Can you work these out from the model? Positions are in its coordinate system, mm. A direction names the side the tool comes from. Give positions to 0.01 mm unless a question says otherwise; leave off trailing zeros. Answer as CSV lines item,"result".
```python
from build123d import *

# Parameters (mm, degrees)
F1_DEPTH  = 6.35
F2_DEPTH  = 3.175
F3_DEPTH  = 2.8222222222
F4_DEPTH  = 2.4694444444
F5_DEPTH  = 2.4694444444
F6_DEPTH  = 2.1166666667
F7_DEPTH  = 1.4111111111
F8_DEPTH  = 1.0583333333
F9_DEPTH  = 0.3527777778
F10_DEPTH = 0.7055555556
F12_DEPTH = 2.54
F13_R     = 2.38125
F14_DEPTH = 25.4
F15_R     = 2.53999
F16_R     = 2.53999
F18_DEPTH = 2.54


# Not quite as in the source:
# - a fillet or chamfer is up to 0.001 mm smaller than in the source, because OpenCascade refuses the exact size


with BuildPart() as f1:
    # F0 (on Top) → F1 (new body)
    with BuildSketch(Plane.XY):
        Polygon((152.4, 3.6661742094), (152.4, 0), (152.4, -3.6661742094), (158.75, -7.3323484187), (165.1, -3.6661742094), (165.1, 3.6661742094), (158.75, 7.3323484187), align=None)
    extrude(amount=F1_DEPTH)

    # F6 (add): a face of the model
    f6_faces = [f1.faces().sort_by_distance(p)[0] for p in [
        (158.75, 0, 6.35),
    ]]
    extrude(f6_faces, amount=F6_DEPTH)


with BuildPart() as f1b:
    # F0 (on Top) → F1, piece 2 (new body)
    with BuildSketch(Plane.XY):
        Polygon((144.4625, -36.2669128953), (141.2875, -34.4338257906), (138.1125, -36.2669128953), (138.1125, -39.9330871047), (141.2875, -41.7661742094), (144.4625, -39.9330871047), align=None)
    extrude(amount=F1_DEPTH)


with BuildPart() as f1c:
    # F0 (on Top) → F1, piece 3 (new body)
    with BuildSketch(Plane.XY):
        Polygon((116.68125, 4.1244459855), (116.68125, 0), (123.825, 0), (130.96875, 0), (130.96875, 4.1244459855), (123.825, 8.248891971), align=None)
        Polygon((123.825, 0), (116.68125, 0), (116.68125, -4.1244459855), (123.825, -8.248891971), (130.96875, -4.1244459855), (130.96875, 0), align=None)
    extrude(amount=F1_DEPTH)

    # F5 (add): a face of the model
    f5_faces = [f1c.faces().sort_by_distance(p)[0] for p in [
        (123.825, 0, 6.35),
    ]]
    extrude(f5_faces, amount=F5_DEPTH)


with BuildPart() as f1d:
    # F0 (on Top) → F1, piece 4 (new body)
    with BuildSketch(Plane.XY):
        Polygon((108.74375, -35.8086411192), (104.775, -33.5172822383), (100.80625, -35.8086411192), (100.80625, -40.3913588808), (104.775, -42.6827177617), (108.74375, -40.3913588808), align=None)
    extrude(amount=F1_DEPTH)

    # F9 (add): a face of the model
    f9_faces = [f1d.faces().sort_by_distance(p)[0] for p in [
        (104.775, -38.1, 6.35),
    ]]
    extrude(f9_faces, amount=F9_DEPTH)


with BuildPart() as f1e:
    # F0 (on Top) → F1, piece 5 (new body)
    with BuildSketch(Plane.XY):
        Polygon((77.7875, 4.5827177617), (77.7875, 0), (85.725, 0), (93.6625, 0), (93.6625, 4.5827177617), (85.725, 9.1654355234), align=None)
        Polygon((85.725, 0), (77.7875, 0), (77.7875, -4.5827177617), (85.725, -9.1654355234), (93.6625, -4.5827177617), (93.6625, 0), align=None)
    extrude(amount=F1_DEPTH)

    # F4 (add): a face of the model
    f4_faces = [f1e.faces().sort_by_distance(p)[0] for p in [
        (85.725, 0, 6.35),
    ]]
    extrude(f4_faces, amount=F4_DEPTH)


with BuildPart() as f1f:
    # F0 (on Top) → F1, piece 6 (new body)
    with BuildSketch(Plane.XY):
        Polygon((69.453125, -35.5795052311), (65.0875, -33.0590104621), (60.721875, -35.5795052311), (60.721875, -40.6204947689), (65.0875, -43.1409895379), (69.453125, -40.6204947689), align=None)
    extrude(amount=F1_DEPTH)

    # F10 (add): a face of the model
    f10_faces = [f1f.faces().sort_by_distance(p)[0] for p in [
        (65.0875, -38.1, 6.35),
    ]]
    extrude(f10_faces, amount=F10_DEPTH)


with BuildPart() as f1g:
    # F0 (on Top) → F1, piece 7 (new body)
    with BuildSketch(Plane.XY):
        Polygon((35.71875, 5.0409895379), (35.71875, 0), (44.45, 0), (53.18125, 0), (53.18125, 5.0409895379), (44.45, 10.0819790757), align=None)
        Polygon((44.45, 0), (35.71875, 0), (35.71875, -5.0409895379), (44.45, -10.0819790757), (53.18125, -5.0409895379), (53.18125, 0), align=None)
    extrude(amount=F1_DEPTH)

    # F3 (add): a face of the model
    f3_faces = [f1g.faces().sort_by_distance(p)[0] for p in [
        (44.45, 0, 6.35),
    ]]
    extrude(f3_faces, amount=F3_DEPTH)


with BuildPart() as f1h:
    # F0 (on Top) → F1, piece 8 (new body)
    with BuildSketch(Plane.XY):
        Polygon((-18.25625, -41.3079024332), (-18.25625, -38.1), (-18.25625, -34.8920975668), (-23.8125, -31.6841951336), (-29.36875, -34.8920975668), (-29.36875, -41.3079024332), (-23.8125, -44.5158048664), align=None)
    extrude(amount=F1_DEPTH)

    # F7 (add): a face of the model
    f7_faces = [f1h.faces().sort_by_distance(p)[0] for p in [
        (-23.8125, -38.1, 6.35),
    ]]
    extrude(f7_faces, amount=F7_DEPTH)


with BuildPart() as f1i:
    # F0 (on Top) → F1, piece 9 (new body)
    with BuildSketch(Plane.XY):
        Polygon((26.9875, -35.350369343), (22.225, -32.600738686), (22.225, -38.1), (17.4625, -38.1), (17.4625, -40.849630657), (22.225, -43.599261314), (26.9875, -40.849630657), align=None)
        Polygon((22.225, -38.1), (22.225, -32.600738686), (17.4625, -35.350369343), (17.4625, -38.1), align=None)
    extrude(amount=F1_DEPTH)

    # F8 (add): a face of the model
    f8_faces = [f1i.faces().sort_by_distance(p)[0] for p in [
        (22.225, -38.1, 6.35),
    ]]
    extrude(f8_faces, amount=F8_DEPTH)


with BuildPart() as f1j:
    # F0 (on Top) → F1, piece 10 (new body)
    with BuildSketch(Plane.XY):
        Polygon((9.525, -5.499261314), (9.525, 0), (9.525, 5.499261314), (0, 10.9985226281), (-9.525, 5.499261314), (-9.525, -5.499261314), (0, -10.9985226281), align=None)
    extrude(amount=F1_DEPTH)

    # F2 (add): a face of the model
    f2_faces = [f1j.faces().sort_by_distance(p)[0] for p in [
        (0, 0, 6.35),
    ]]
    extrude(f2_faces, amount=F2_DEPTH)


with BuildPart() as f12:
    # F11 (on face) → F12 (new body)
    with BuildSketch(Plane(origin=(0, 0, 0), x_dir=(1, 0, 0), z_dir=(0, 0, -1))):
        with BuildLine():
            Line((141.2875, 47.6267617683), (-23.5682692308, 50.7976514101))
            ThreePointArc((-23.5682692308, 50.7976514101), (-14.7463064556, 46.9934883266), (-11.1125, 38.1))
            Line((-11.1125, 38.1), (131.7625, 38.1))
            ThreePointArc((131.7625, 38.1), (134.617383755, 44.8996451583), (141.4706730769, 47.6232385575))
            Line((141.4706730769, 47.6232385575), (141.2875, 47.6267617683))
        make_face()
        with BuildLine():
            Line((-35.4252854215, 32.9586757782), (-17.4191781323, -7.7119863327))
            ThreePointArc((-17.4191781323, -7.7119863327), (-10.2318580693, -16.0689632662), (0.381, -19.0461896189))
            ThreePointArc((0.381, -19.0461896189), (13.6044211564, -13.335), (19.05, 0))
            Line((19.05, 0), (142.875, 0))
            ThreePointArc((142.875, 0), (147.6375, -11.3370176303), (159.0675, -15.8718246824))
            ThreePointArc((159.0675, -15.8718246824), (172.7981495603, -7.3935863375), (172.0126501051, 8.7245479648))
            Line((172.0126501051, 8.7245479648), (149.245090063, 43.3347287789))
            ThreePointArc((149.245090063, 43.3347287789), (145.8881342123, 46.4402511859), (141.4706730769, 47.6232385575))
            ThreePointArc((141.4706730769, 47.6232385575), (134.617383755, 44.8996451583), (131.7625, 38.1))
            Line((131.7625, 38.1), (-11.1125, 38.1))
            ThreePointArc((-11.1125, 38.1), (-14.7463064556, 46.9934883266), (-23.5682692308, 50.7976514101))
            ThreePointArc((-23.5682692308, 50.7976514101), (-34.3892798322, 45.1300589173), (-35.4252854215, 32.9586757782))
        make_face()
        Polygon((9.525, 5.499261314), (9.525, 0), (9.525, -5.499261314), (0, -10.9985226281), (-9.525, -5.499261314), (-9.525, 5.499261314), (0, 10.9985226281), align=None, mode=Mode.SUBTRACT)
        with BuildLine():
            ThreePointArc((19.05, 0), (13.6044211564, -13.335), (0.381, -19.0461896189))
            Line((0.381, -19.0461896189), (159.0675, -15.8718246824))
            ThreePointArc((159.0675, -15.8718246824), (147.6375, -11.3370176303), (142.875, 0))
            Line((142.875, 0), (19.05, 0))
        make_face()
    extrude(amount=F12_DEPTH)

    # F13 (on face) → F14 (cut)
    with BuildSketch(Plane(origin=(0, 0, -2.54), x_dir=(1, 0, 0), z_dir=(0, 0, -1))):
        with Locations((22.225, 19.900738686)):
            Circle(F13_R)
        with Locations((123.825, 19.900738686)):
            Circle(F13_R)
    extrude(amount=-F14_DEPTH, mode=Mode.SUBTRACT)

    # F15 (radius 2.54 in the source; OpenCascade refuses exactly that, so slightly less here)
    f15_edges = [f12.edges().sort_by_distance(p)[0] for p in [
        (19.84375, -19.900739, 0),
    ]]
    fillet(f15_edges, radius=F15_R)

    # F16 (radius 2.54 in the source; OpenCascade refuses exactly that, so slightly less here)
    f16_edges = [f12.edges().sort_by_distance(p)[0] for p in [
        (58.951202, -49.210445, 0),
        (121.44375, -19.900739, 0),
    ]]
    fillet(f16_edges, radius=F16_R)


with BuildPart() as f1j_1:
    add(f1j.part)

    # F17: union F1g, F1e, F1c, F1, F1h, F1i, F1f, F1d, F1b, F12
    add(f1g.part)
    add(f1e.part)
    add(f1c.part)
    add(f1.part)
    add(f1h.part)
    add(f1i.part)
    add(f1f.part)
    add(f1d.part)
    add(f1b.part)
    add(f12.part)

    # F18 (add, through all): a face of the model
    f18_faces = [f1j_1.faces().sort_by_distance(p)[0] for p in [
        (0, 0, 0),
    ]]
    extrude(f18_faces, amount=F18_DEPTH)


solid = f1j_1.part
```
Item 1: Please list where these lines run through material, in increasing order: line 1 along X through (y, z) = (9, 8); line 2 along X through (y, z) = (-36, 3.25); line 3 along X through (y, z) = (2.5, 0.25) (1 decimal).
Numbers:
line 1,"x = -3.46 to 3.46, 42.58 to 46.32, 85.44 to 86.01"
line 2,"x = -29.37 to -18.26, 17.46 to 26.99, 60.72 to 69.45, 100.81 to 108.74, 138.57 to 144"
line 3,"x = -9.5 to 9.5, 35.7 to 53.2, 77.8 to 93.7, 116.7 to 131, 152.4 to 165.1"
Item 2: For pin 1 (6 mm diameter, centred on y = -38.5, z = 4.5, fed in from +X); pin 2 (12 mm diameter, centred on x = 44.5, y = -16, fed in from +Z); pin 3 (6.5 mm diameter, centred on x = 103, y = -40, fed in from +Z), each with a flat end and sliding along its axis, tell me the tip position at first contact or that it passes through.
Numbers:
pin 1,"stops at x = 144.46"
pin 2,"stops at z = 9.17"
pin 3,"stops at z = 6.7"
Item 3: We'd pull the mould along X, two halves only. Please class faces 6 (the cylindrical face through (-25.598, -12.648, -0.724)), 7 (the flat face through (19.8, -42.2, 3.7)), 8 (the flat face through (105, -38, 6.703)): released by +X, released by -X, zero draft, split by the parting line, or undercut.
Numbers:
face 6,"released by -X"
face 7,"undercut"
face 8,"zero draft"
Item 4: Imagine slicing it at A-A, the plane z = 3.5. Give the number of separate pieces and of enclosed holes in the cut face, then the cut area to 3 significant figures.
Numbers:
separate pieces,"10"
enclosed holes,"0"
area,"1,450 mm²"
Item 5: For faces 1 (the flat face through (-21.073, -42.934, 3.826)), 2 (the flat face through (152.4, 0, 4)), 3 (the flat face through (-29.369, -38, 4)), 4 (the flat face through (102.818, -34.647, 3.304)), 5 (the flat face through (144.462, -38, 3)), which set-ups out of +Z, -Z, +X, -X, +Y, -Y let a thin tool reach every point of the face, with its end or its side?
Numbers:
face 1,"+Z, -Y"
face 2,"+Z, +Y, -Y"
face 3,"+Z, -X, +Y, -Y"
face 4,"+Z, +Y"
face 5,"+Z, +X, +Y, -Y"
